Design review of the part built by this model. Coordinates are the model's own, in mm. Face numbers are marked on the shaded views. A direction names the side the tool comes from. Give positions to 0.01 mm unless a question says otherwise; leave off trailing zeros. Loops run counter-clockwise (first coordinate to the right, second up) from the corner with the lowest first, then second, coordinate; pieces in that order, holes last. Notation, with made-up numbers: (-14.5, 20) -> (17.5, 20) arc R18 ccw to (17.5, 42) -> close; hole circle Ø2 at (-29, 40.25). An arc over 180 degrees is marked (long way). Use CSV: the item, a comma, the result in double quotes. Start each with the question number.
Item 1: Wall thickness on line 1 along X through (y, z) = (3.5, 15.5); line 2 along Z through (x, y) = (17, 0.5); line 3 along X through (y, z) = (7, 21): over which ranges is each line inside the solid? List them lowest first. Write a range as from..to.
Item 2: We need section A-A (y = 5.25). State the section outline as (x, z) points, plus the area to 3 significant figures.
Item 3: We need section C-C (x = 23.5). State the section outline as (y, z) points (3 decimals).
Item 4: The part is to be moulded in two halves that separate along X. For the marked faces 3, 4 and 5, say which applies: +X half, -X half, draft (parallel to the pull), parting line (faces both ways), or undercut.
Item 5: We need section D-D (y = 0). State the section outline as (x, z) points (3 decimals).
Item 6: We need section B-B (z = 30). State the section outline as (x, y) points (3 decimals), plus the area to 3 significant figures.
Item 7: Clearance check with flat-ended pins moving along their axes: pin 1 (6 mm diameter, centred on x = -7, z = -1, fed in from -Y) (3 decimals); pin 2 (4 mm diameter, centred on x = -21.5, y = -4.5, fed in from -Z); pin 3 (1 mm diameter, centred on x = -45.5, z = 21.5, fed in from +Y); pin 4 (6 mm diameter, centred on y = -5, z = 52, fed in from +X). State where each tip first meets the part, or that it passes through.
Item 8: For the marked faces 1 and 2, list the 3-axis set-ups (+Z, -Z, +X, -X, +Y, -Y) from which the entire face can be reached by the end or side of a thin tool; tool diameter is ignored.
from build123d import *

# Parameters (mm, degrees)
SKETCH3_R           = 9.525
BOSS_EXTRUDE1_DEPTH = 63.5
SKETCH4_R           = 6.35
BOSS_EXTRUDE2_DEPTH = 63.5


with BuildPart() as part:
    # Sketch3 → Boss-Extrude1 (new body, symmetric)
    with BuildSketch(Plane(origin=(0, 0, 0), x_dir=(0, 0, -1), z_dir=(1, 0, 0))):
        Circle(SKETCH3_R)
    extrude(amount=BOSS_EXTRUDE1_DEPTH, both=True)

    # Sketch4 → Boss-Extrude2 (add)
    with BuildSketch(Plane.XY):
        with Locations((-37.967477859, 3.175)):
            Circle(SKETCH4_R)
        with Locations((38.232522141, 3.175)):
            Circle(SKETCH4_R)
    extrude(amount=BOSS_EXTRUDE2_DEPTH)


solid = part.part
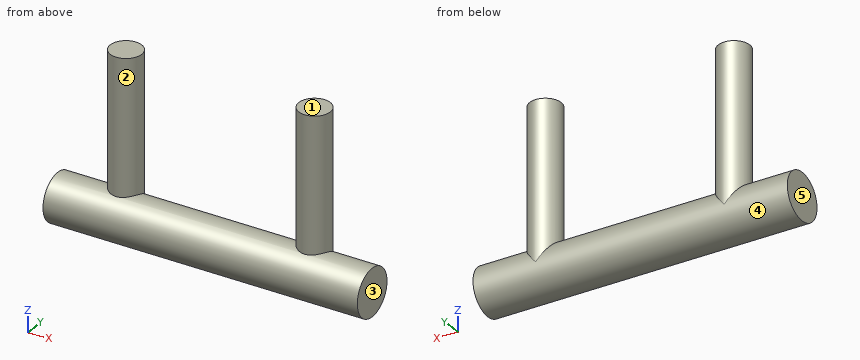
Results found:
1,line 1,"-44.31..-31.63, 31.89..44.57"
1,line 2,"-9.51..9.51"
1,line 3,"-43.04..-32.9, 33.16..43.3"
2,outline,"(-63.5, -7.95) -> (63.5, -7.95) -> (63.5, 7.95) -> (44.23, 7.95) -> (44.23, 63.5) -> (32.23, 63.5) -> (32.23, 7.95) -> (-31.97, 7.95) -> (-31.97, 63.5) -> (-43.97, 63.5) -> (-43.97, 7.95) -> (-63.5, 7.95) -> close"
2,area,"3,350 mm²"
3,outline,"circle Ø19.05 at (0, 0)"
4,face 3,"+X half"
4,face 4,"undercut"
4,face 5,"-X half"
5,outline,"(-63.5, -9.525) -> (63.5, -9.525) -> (63.5, 9.525) -> (43.732, 9.525) -> (43.732, 63.5) -> (32.733, 63.5) -> (32.733, 9.525) -> (-32.468, 9.525) -> (-32.468, 63.5) -> (-43.467, 63.5) -> (-43.467, 9.525) -> (-63.5, 9.525) -> close"
6,outline,"circle Ø12.7 at (-37.967, 3.175); circle Ø12.7 at (38.233, 3.175)"
6,area,"253 mm²"
7,pin 1,"y = -9.525"
7,pin 2,"z = -9.19"
7,pin 3,"through"
7,pin 4,"x = 41.91"
8,face 1,"+Z, +X, -X, +Y, -Y"
8,face 2,"+Z"
